Geometry: see drawing. Coordinates: mm, zero at the bounding-box minimum. A direction names the side the tool comes from. Give positions to 0.01 mm unless a question says otherwise; leave off trailing zeros. Write each loop counter-clockwise with the first axis right and the second up, starting at its lowest first coordinate (ties: lowest second). Pieces come first, ordered by that corner, then holes. Notation, with made-up numbers: (-6, -35) -> (22, -35) arc R27 ccw to (22, -11) -> close; hole circle Ø3 at (50, -19.5). An arc over 180 degrees is marked (long way). Answer as a JSON object with one key per item and string values. Group by question number.
Item 1: Ray query, probe 1 along Z at (x, y) = (46.5, 77); probe 2 along Y at (x, z) = (98, 45) (1 decimal); probe 3 along X at (y, z) = (109, 13). Return the intervals inside material, ascending. Write a range as from..to.
Item 2: Pull-direction query (Y, two-part tool) for the marked faces 4, 5 and 6; classes: pulls with the +Y half, pulls with the -Y half, needs draft (parallel to the pull), parting line crosses it, or undercut.
Item 3: Section query D-D on x = 114.5. Return the cut outline in (y, z) (1 decimal).
Item 4: First-contact query: pin 1 Ø4 at (y, z) = (105, 63.5) entering from +X; pin 2 Ø3 at (x, y) = (106.5, 73.5) entering from +Z; pin 3 Ø6 at (x, y) = (83.5, 80.5) entering from +Z; pin 4 Ø1.5 at (y, z) = (113, 93) entering from -X. Flat tips, straight axial feed; report the tip coordinate or a pass-through.
Item 5: Section query C-C on x = 87. Return the cut outline in (y, z) (1 decimal).
Item 6: Access query for the marked faces 1, 2 and 3. Directions: +Z, -Z, +X, -X, +Y, -Y. A direction counts if a zero-diameter tool reaches every point of the face in a straight line with its end or side. Return the directions, or none.
Item 7: Section query A-A on z = 52. Return the cut outline in (x, y) (1 decimal).
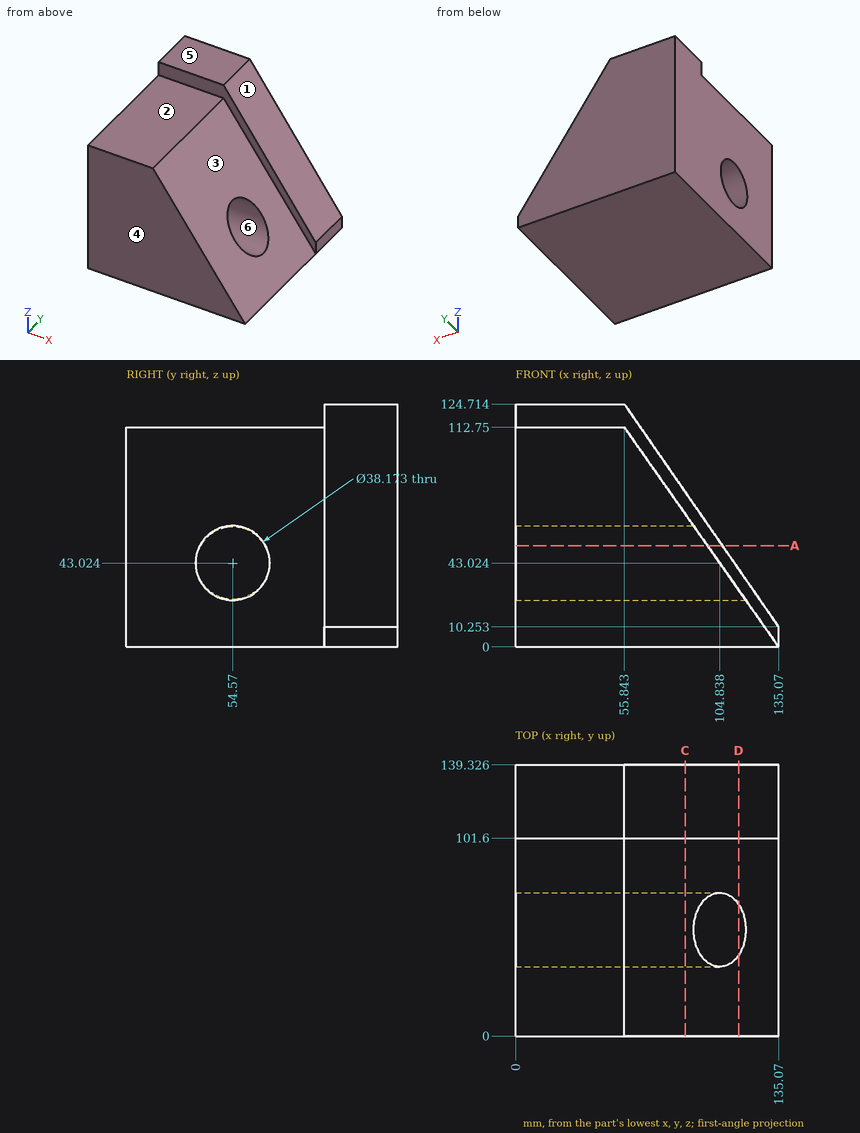
Worked answers:
{
 "1": {"probe 1": "0..112.75", "probe 2": "0..35.6, 73.6..139.3", "probe 3": "0..133.17"},
 "2": {"face 4": "pulls with the -Y half", "face 5": "needs draft", "face 6": "undercut"},
 "3": {"outline": "(0, 0) -> (139.3, 0) -> (139.3, 40) -> (101.6, 40) -> (101.6, 29.3) -> (67.8, 29.3) arc R19.1 cw to (41.3, 29.3) -> (0, 29.3) -> close"},
 "4": {"pin 1": "x = 99.6", "pin 2": "z = 42.78", "pin 3": "z = 77.66", "pin 4": "x = 0"},
 "5": {"outline": "(0, 0) -> (139.3, 0) -> (139.3, 79.7) -> (101.6, 79.7) -> (101.6, 68.4) -> (0, 68.4) -> close; hole circle Ø38.2 at (54.6, 43)"},
 "6": {"face 1": "+Z, +X, +Y, -Y", "face 2": "+Z, +X, -X, -Y", "face 3": "+Z, +X, -Y"},
 "7": {"outline": "(0, 0) -> (98.5, 0) -> (98.5, 37.7) -> (0, 37.7) -> close; (0, 71.4) -> (98.5, 71.4) -> (98.5, 101.6) -> (106.2, 101.6) -> (106.2, 139.3) -> (0, 139.3) -> close"}
}
